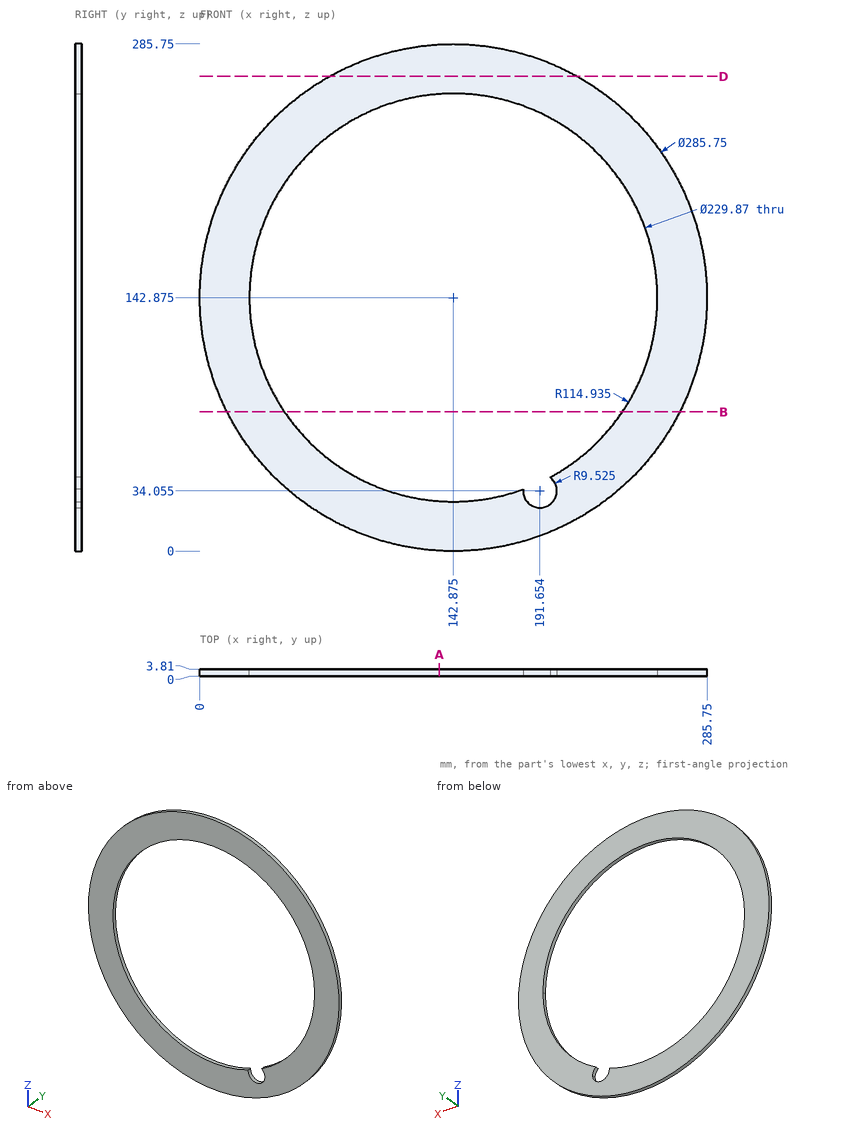
Drawing for the job (mm, zero at the part's lowest x, y, z). Round coordinates to 2 decimals unless told otherwise and drop trailing zeros. Order: outer loops, then holes, each group sorted by start corner. A loop starts at its lowest first (then second) coordinate and runs counter-clockwise, first axis right, second up. Notation, with made-up numbers: (88.5, 8) -> (121.5, 8) arc R24 ccw to (121.5, 42) -> close; hole circle Ø3 at (57, -26.5). An arc over 180 degrees is marked (long way). Put each result on its own line as item: value.
Q1. Band-saw the part on B-B (z = 78.5). Give the cut face in (x, y) (1 decimal).
From the geometry:
outline: (15.3, 0) -> (47.7, 0) -> (47.7, 3.8) -> (15.3, 3.8) -> close; (238.1, 0) -> (270.4, 0) -> (270.4, 3.8) -> (238.1, 3.8) -> close
Q2. Wall check: line 1 (Z direction, x = 190, y = 0.35) (1 decimal); line 2 (Z direction, x = 66.5, y = 0.2) (1 decimal); line 3 (X direction, y = 2.65, z = 233.5) (1 decimal). Give the ranges that are in metal, low to high. Write a range as [from, to].
From the geometry:
line 1: z = [8, 24.7], [247.7, 277.8]
line 2: z = [22.1, 57], [228.8, 263.6]
line 3: x = [32.4, 72.2], [213.6, 253.3]
Q3. Pin check, flat tips, straight feed: pin 1 Ø1 at (x, y) = (134, 2) entering from -Z; pin 2 Ø2 at (y, z) = (2.5, 162.5) entering from -X; pin 3 Ø1 at (x, y) = (152, 2) entering from -Z. Stop position of each tip, or through.
From the geometry:
pin 1: stops at z = 0.25
pin 2: stops at x = 1.22
pin 3: stops at z = 0.26
Q4. Band-saw the part on D-D (z = 267.5). Give the cut face in (x, y) (1 decimal).
From the geometry:
outline: (73, 0) -> (212.7, 0) -> (212.7, 3.8) -> (73, 3.8) -> close
Q5. Band-saw the part on A-A (x = 135). Give the cut face in (y, z).
From the geometry:
outline: (0, 0.22) -> (3.81, 0.22) -> (3.81, 28.21) -> (0, 28.21) -> close; (0, 257.54) -> (3.81, 257.54) -> (3.81, 285.53) -> (0, 285.53) -> close
